Autodesk Inventor part; units mm, degrees
ref_plane "YZ Plane" through (0, 0, 0) normal (1, 0, 0) x (0, 1, 0)
ref_plane "XZ Plane" through (0, 0, 0) normal (0, 1, 0) x (-1, 0, 0)
ref_plane "XY Plane" through (0, 0, 0) normal (0, 0, 1) x (1, 0, 0)
sketch "Sketch1" plane through (0, 0, 0) normal (0, 1, 0) x (-1, 0, 0)
  line L0 (0, 0) -> (65, 0)
  line L1 (65, 0) -> (65, -70.6)
  line L2 (65, -70.6) -> (0, -70.6)
  line L3 (0, -70.6) -> (0, 0)
  line L4 (30, -12.6) -> (12.6, -12.6)
  line L5 (12.6, -12.6) -> (12.6, -58)
  line L6 (12.6, -58) -> (30, -58)
  line L7 (30, -58) -> (30, -12.6)
  dimension "d0" = 70.6
  dimension "d1" = 65
  dimension "d2" = 45.4
  dimension "d3" = 17.4
  dimension "d4" = 12.6
  dimension "d5" = 12.6
extrude "Extrusion1" add sketch "Sketch1" along normal blind 5
sketch "Sketch2" plane through (0, 5, 0) normal (0, 1, 0) x (1, 0, 0)
  line L0 (-12.6, 58) -> (-12.6, 12.6) construction
  line L1 (-12.6, 12.6) -> (0, 12.6) construction
  line L2 (0, 0) -> (0, 70.6) construction
  line L3 (-6.3, 6.3) -> (-6.3, 12.6) construction
  line L4 (-12.6, 12.6) -> (-30, 12.6) construction
  line L5 (-12.6, 12.6) -> (-12.6, 0) construction
  line L6 (-65, 0) -> (0, 0) construction
  line L7 (-6.3, 6.3) -> (-12.6, 6.3) construction
  line L8 (-6.3, 6.3) -> (-36.3, 6.3) construction
  line L9 (-36.3, 6.3) -> (-36.3, 64.3) construction
  line L10 (-36.3, 64.3) -> (-6.3, 64.3) construction
  line L11 (-6.3, 64.3) -> (-6.3, 6.3) construction
  line L12 (-6.3, 64.3) -> (-6.3, 70.6) construction
  line L13 (0, 70.6) -> (-65, 70.6) construction
  line L14 (-36.3, 35.3) -> (-30, 35.3) construction
  line L15 (-30, 12.6) -> (-30, 58) construction
hole "Hole1" at (-36.3, 5, -6.3) at (-6.3, 5, -6.3) at (-36.3, 5, -64.3) at (-6.3, 5, -64.3) direction (0, -1, 0) diameter 6.3 depth 5
sketch "Sketch3" plane through (0, 5, 0) normal (0, 1, 0) x (1, 0, 0)
  circle A0 centre (-6.3, 6.3) radius 3.15
  circle A1 centre (-6.3, 6.3) radius 4.15
  circle A2 centre (-36.3, 6.3) radius 3.15
  circle A3 centre (-36.3, 6.3) radius 4.15
  circle A4 centre (-36.3, 64.3) radius 3.15
  circle A5 centre (-36.3, 64.3) radius 4.15
  circle A6 centre (-6.3, 64.3) radius 3.15
  circle A7 centre (-6.3, 64.3) radius 4.15
  point P0 (0, 0)
  dimension "d15" = 1
extrude "Extrusion2" add sketch "Sketch3" along normal blind 5
sketch "Sketch4" plane through (0, 5, 0) normal (0, 1, 0) x (1, 0, 0)
  circle A0 centre (-36.3, 6.3) radius 4.15 construction
  circle A1 centre (-36.3, 64.3) radius 3.15 construction
  line L0 (-36.3, 6.3) -> (-36.3, 64.3) construction
  line L1 (-36.3, 64.3) -> (-6.3, 64.3) construction
  circle A2 centre (-6.3, 6.3) radius 3.15 construction
  line L2 (-36.3, 6.3) -> (-6.3, 6.3) construction
  circle A3 centre (-6.3, 64.3) radius 3.15 construction
  line L3 (-6.3, 6.3) -> (-6.3, 64.3) construction
  line L4 (-36.3, 35.3) -> (-6.3, 35.3) construction
  line L5 (-36.3, 20.8) -> (-6.3, 20.8) construction
  line L6 (-36.3, 49.8) -> (-6.3, 49.8) construction
  point P0 (0, 0)
  point P1 (-21.3, 64.3)
  point P2 (-21.3, 6.3)
  dimension "d18" = 14.5
hole "Hole2" at (-36.3, 5, -20.8) at (-36.3, 5, -49.8) at (-6.3, 5, -20.8) at (-6.3, 5, -49.8) at (-21.3, 5, -64.3) at (-21.3, 5, -6.3) direction (0, -1, 0) diameter 3 depth 5
equation "\"d0\" = carriage_mount_width"
equation "\"d1\" = carriage_mount_length"
equation "\"d2\" = carriage_mount_cutout_length"
equation "\"d3\" = carriage_mount_cutout_width"
equation "\"d4\" = 0.5 * carriage_mount_width - 0.5 * carriage_mount_cutout_length"
equation "\"d5\" = 0.5 * carriage_mount_width - 0.5 * carriage_mount_cutout_length"
equation "\"d6\" = carriage_mount_thickness"
equation "\"d8\" = rod_diameter + rod_tolerance"
equation "\"d15\" = carriage_mount_wall_thickness"
equation "\"d16\" = carriage_mount_thickness"
equation "\"d18\" = 0.125 * carriage_mount_cutout_length + 0.125 * carriage_mount_width"
equation "\"d19\" = screw_diameter"
equation "\"carriage_mount_length\" = 65"
equation "\"carriage_mount_width\" = 70.6"
equation "\"carriage_mount_cutout_length\" = 45.4"
equation "\"carriage_mount_cutout_width\" = 17.4"
equation "\"screw_diameter\" = 3"
equation "\"rod_diameter\" = 6"
equation "\"rod_tolerance\" = 0.3"
equation "\"carriage_mount_wall_thickness\" = 1"
equation "\"carriage_mount_thickness\" = 5"
properties part number "carriage_mount"
Check sheet for the modelled part. Datum: model origin and axes. Units: mm. A direction names the side the tool comes from. Round coordinates to 2 decimals unless told otherwise and drop trailing zeros. Order: outer loops, then holes, each group sorted by start corner. A loop starts at its lowest first (then second) coordinate and runs counter-clockwise, first axis right, second up.
1) Section check D-D (y = 3.5). Give the number of separate pieces and of enclosed holes in the cut face, and give its area (3 significant figures).
2) Scan lines: line 1 (X direction, y = 3.25, z = -64.3); line 2 (Z direction, x = -21.3, y = 2.85); line 3 (Z direction, x = -36.3, y = 1.95). Record each from-to range of solid material in increasing order.
3) Section check C-C (x = -16). Record the boundary of the cut face in (y, z).
4) Go/stop test with flat-tipped pins: pin 1 Ø4 at (x, y) = (-33.5, 7.5) entering from -Z; pin 2 Ø2.5 at (x, z) = (-6.3, -20.8) entering from -Y; pin 3 Ø8 at (x, z) = (-12, -48) entering from -Y; pin 4 Ø4 at (x, z) = (-21.3, -6.3) entering from +Y. Record where each tip stops, or that it passes through.
5) Section check A-A (y = 8.5). Record the boundary of the cut face in (x, z).
6) Tool access check on faces 1 (the flat face through (-30, 2, -36)), 2 (the flat face through (0, 2, -36)), 3 (the cylindrical face through (-4.385, 7.465, -9.982)). Record the directions out of +Z, -Z, +X, -X, +Y, -Y that give a thin tool (end or side, any length) a straight path to the whole face; none if there is none.
7) Section check B-B (z = -20.8). Record the boundary of the cut face in (x, y).
8) Mould release check, pull along Z, two halves, no side actions. Record for faces 4 (the flat face through (-33, 2, -70.6)), 5 (the flat face through (-32, 5, -35)), 6 (the flat face through (-65, 2, -35)): +Z half, -Z half, draft (parallel to the pull), parting line (faces both ways), or undercut.
Result:
1. separate pieces: 1
1. enclosed holes: 11
1. area: 3,630 mm2
2. line 1: x = -65 to -39.45, -33.15 to -22.8, -19.8 to -9.45, -3.15 to 0
2. line 2: z = -70.6 to -65.8, -62.8 to -58, -12.6 to -7.8, -4.8 to 0
2. line 3: z = -70.6 to -67.45, -61.15 to -51.3, -48.3 to -22.3, -19.3 to -9.45, -3.15 to 0
3. outline: (0, -70.6) - (5, -70.6) - (5, -58) - (0, -58) - close; (0, -12.6) - (5, -12.6) - (5, 0) - (0, 0) - close
4. pin 1: stops at z = -68.37
4. pin 2: passes through
4. pin 3: stops at y = 0
4. pin 4: stops at y = 5
5. outline: circle Ø8.3 at (-36.3, -64.3); circle Ø8.3 at (-36.3, -6.3); circle Ø8.3 at (-6.3, -64.3); circle Ø8.3 at (-6.3, -6.3); hole circle Ø6.3 at (-36.3, -64.3); hole circle Ø6.3 at (-36.3, -6.3); hole circle Ø6.3 at (-6.3, -64.3); hole circle Ø6.3 at (-6.3, -6.3)
6. face 1: +Y, -Y
6. face 2: +Z, -Z, +X, +Y, -Y
6. face 3: +Y
7. outline: (-65, 0) - (-37.8, 0) - (-37.8, 5) - (-65, 5) - close; (-34.8, 0) - (-30, 0) - (-30, 5) - (-34.8, 5) - close; (-12.6, 0) - (-7.8, 0) - (-7.8, 5) - (-12.6, 5) - close; (-4.8, 0) - (0, 0) - (0, 5) - (-4.8, 5) - close
8. face 4: -Z half
8. face 5: undercut
8. face 6: draft
